Design review of the part built by this model. Coordinates are the model's own, in mm. A direction names the side the tool comes from. Give positions to 0.01 mm unless a question says otherwise; leave off trailing zeros. Loops run counter-clockwise (first coordinate to the right, second up) from the corner with the lowest first, then second, coordinate; pieces in that order, holes last. Notation, with made-up numbers: (26.25, 51.25) -> (55.25, 51.25) arc R35 ccw to (55.25, 83.25) -> close; hole circle Ø1 at (75.25, 69). An arc over 180 degrees is marked (long way). Use CSV: the item, a comma, the result in double quotes. Start each with the question number.
Item 1: Wall thickness on line 1 along Y through (x, z) = (-6, -20); line 2 along Y through (x, z) = (13, 21); line 3 along Y through (x, z) = (-3, 9): over which ranges is each line inside the solid? List them lowest first. Write a range as from..to.
Item 2: We need section B-B (x = 0). State the section outline as (y, z) points.
Item 3: The part is to be moulded in two halves that separate along Z. For faces 4 (the face through (36.81, 1.52, 15.54)), 5 (the face through (50, 8, 0)), 6 (the face through (1, -3, 32.5)), say which applies: +Z half, -Z half, draft (parallel to the pull), parting line (faces both ways), or undercut.
Item 4: We need section C-C (y = -32). State the section outline as (x, z) points, plus the area to 3 significant figures.
Item 5: We need section D-D (x = 28.5). State the section outline as (y, z) points, plus the area to 4 significant figures.
Item 6: For faces 1 (the face through (-42.43, 2, -20.1)), 2 (the face through (-13.17, -17.57, 20.66)), 3 (the face through (-36, 6, 0)), list the 3-axis set-ups (+Z, -Z, +X, -X, +Y, -Y) from which the entire face can be reached by the end or side of a thin tool; tool diameter is ignored.
Item 7: We need section A-A (z = 0). State the section outline as (x, y) points.
Item 8: Clearance check with flat-ended pins moving along their axes: pin 1 (10 mm diameter, centred on x = 5, z = -23, fed in from -Y); pin 2 (1.5 mm diameter, centred on x = -8.5, z = 22, fed in from -Y); pin 3 (10 mm diameter, centred on y = -20, z = 3.5, fed in from +X); pin 4 (1.5 mm diameter, centred on y = -36, z = -14, fed in from +X). State where each tip first meets the part, or that it passes through.
from build123d import *

# Parameters (mm, degrees)
SALIENTE_EXTRUIR1_DEPTH                     = 32.5
REFRENTADO_PARA_TORNILLO_CON_CABEZA_2_COUNT = 2
REFRENTADO_PARA_TORNILLO_CON_CABEZA_2_PITCH = 40


with BuildPart() as part:
    # Croquis2 → Saliente-Extruir1 (new body, symmetric)
    with BuildSketch(Plane.XY):
        Polygon((-30, 0), (30, 0), (42.5, 12.5), (50, 12.5), (50, 2.5), (35, -12.5), (-35, -12.5), (-50, 2.5), (-50, 12.5), (-42.5, 12.5), align=None)
    extrude(amount=SALIENTE_EXTRUIR1_DEPTH, both=True)

    # Croquis3 → Revolución1 (revolve)
    with BuildSketch(Plane.XY):
        Polygon((0, -12.5), (-24.5, -12.5), (-24.5, -22.5), (-19.5, -22.5), (-20, -30.484359711), (-24.5, -30.484359711), (-24.5, -39.5), (-21.5, -42.5), (0, -42.5), align=None)
    revolve(axis=Axis((0, -42.5, 0), (0, 1, 0)))

    # Croquis5 → Refrentado para tornillo con cabeza plana de M81 (revolve, cut)
    with BuildSketch(Plane(origin=(-42.5, -5, -20), x_dir=(0.707106781, -0.707106781, 0), z_dir=(0, 0, 1))):
        Polygon((0, 0), (0, 77.781745931), (4.5, 77.781745931), (4.5, 5), (7.5, 5), (7.5, 0), align=None)
    refrentado_para_tornillo_con_cabeza_plan = revolve(axis=Axis((-46.990128061, -9.490128061, -20), (0.707106781, 0.707106781, 0)), mode=Mode.SUBTRACT)

    # Refrentado para tornillo con cabeza  2: Refrentado para tornillo con cabeza plana de M81 ×2
    with Locations(*[(0, 0, i * REFRENTADO_PARA_TORNILLO_CON_CABEZA_2_PITCH) for i in range(1, REFRENTADO_PARA_TORNILLO_CON_CABEZA_2_COUNT)]):
        add(refrentado_para_tornillo_con_cabeza_plan, mode=Mode.SUBTRACT)

    # Simetría1: Refrentado para tornillo con cabeza plana de M81 across plane
    add(refrentado_para_tornillo_con_cabeza_plan.mirror(Plane(origin=(0, 0, 0), x_dir=(0, 0, 1), z_dir=(1, 0, 0))), mode=Mode.SUBTRACT)

    # Simetría1 copy 1 sketch → Simetría1 copy 1 (revolve, cut)
    with BuildSketch(Plane(origin=(42.5, -5, 20), x_dir=(-0.707106781, -0.707106781, 0), z_dir=(0, 0, 1))):
        Polygon((0, 0), (0, -77.781745931), (4.5, -77.781745931), (4.5, -5), (7.5, -5), (7.5, 0), align=None)
    revolve(axis=Axis((46.990128061, -9.490128061, 20), (0.707106781, -0.707106781, 0)), mode=Mode.SUBTRACT)


solid = part.part
Results found:
1,line 1,"-42.5..-30.48, -22.5..0"
1,line 2,"-12.5..0"
1,line 3,"-42.5..0"
2,outline,"(-42.5, -21.5) -> (-39.5, -24.5) -> (-30.48, -24.5) -> (-30.48, -20) -> (-22.5, -19.5) -> (-22.5, -24.5) -> (-12.5, -24.5) -> (-12.5, -32.5) -> (0, -32.5) -> (0, 32.5) -> (-12.5, 32.5) -> (-12.5, 24.5) -> (-22.5, 24.5) -> (-22.5, 19.5) -> (-30.48, 20) -> (-30.48, 24.5) -> (-39.5, 24.5) -> (-42.5, 21.5) -> close"
3,face 4,"undercut"
3,face 5,"draft"
3,face 6,"+Z half"
4,outline,"circle Ø49 at (0, 0)"
4,area,"1,890 mm²"
5,outline,"(-12.5, -32.5) -> (0, -32.5) -> (0, 32.5) -> (-12.5, 32.5) -> close"
5,area,"812.5 mm²"
6,face 1,"none"
6,face 2,"-Y"
6,face 3,"+Z, -Z, +Y"
7,outline,"(-50, 2.5) -> (-35, -12.5) -> (-24.5, -12.5) -> (-24.5, -22.5) -> (-19.5, -22.5) -> (-20, -30.48) -> (-24.5, -30.48) -> (-24.5, -39.5) -> (-21.5, -42.5) -> (21.5, -42.5) -> (24.5, -39.5) -> (24.5, -30.48) -> (20, -30.48) -> (19.5, -22.5) -> (24.5, -22.5) -> (24.5, -12.5) -> (35, -12.5) -> (50, 2.5) -> (50, 12.5) -> (42.5, 12.5) -> (30, 0) -> (-30, 0) -> (-42.5, 12.5) -> (-50, 12.5) -> close"
8,pin 1,"y = -42.5"
8,pin 2,"y = -41.17"
8,pin 3,"x = 24.5"
8,pin 4,"x = 20.61"
